```python
from build123d import *

# Parameters (mm, degrees)
EXTRUDE_THIN1_DEPTH = 76.2


with BuildPart() as part:
    # Sketch1 → Extrude-Thin1 (new body)
    with BuildSketch(Plane.XY):
        with BuildLine():
            Line((-171.530725158, -169.540176263), (-57.207776809, -14.493356815))
            ThreePointArc((-57.207776809, -14.493356815), (-48.029088686, -5.258412911), (-36.568222458, 0.920668726))
            Line((-36.568222458, 0.920668726), (143.952557391, 66.301099815))
            ThreePointArc((143.952557391, 66.301099815), (253.095507904, 33.210999285), (252.264699452, -80.834816757))
            Line((252.264699452, -80.834816757), (229.469051384, -110.874685447))
            Line((229.469051384, -110.874685447), (226.93983158, -108.955395947))
            Line((226.93983158, -108.955395947), (249.735479648, -78.915527258))
            ThreePointArc((249.735479648, -78.915527258), (250.538594484, 31.328761583), (145.033742323, 63.315858762))
            Line((145.033742323, 63.315858762), (-35.487037526, -2.064572327))
            ThreePointArc((-35.487037526, -2.064572327), (-46.129270453, -7.80229099), (-54.652337995, -16.377596044))
            Line((-54.652337995, -16.377596044), (-168.975286345, -171.424415492))
            Line((-168.975286345, -171.424415492), (-171.530725158, -169.540176263))
        make_face()
    extrude(amount=EXTRUDE_THIN1_DEPTH)


solid = part.part
```
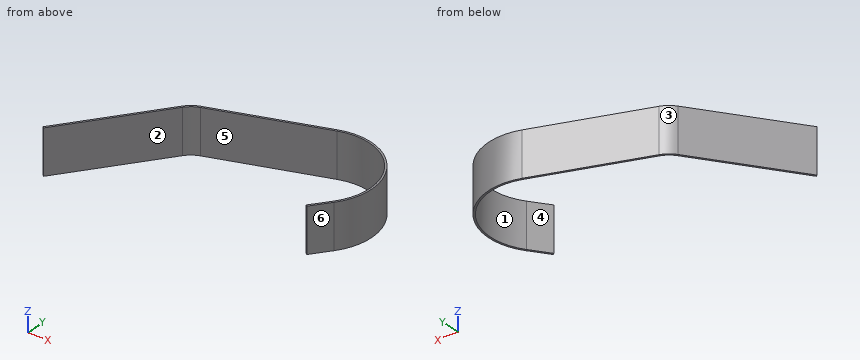
Design review of the part built by this model. Coordinates are the model's own, in mm. Face numbers are marked on the shaded views. A direction names the side the tool comes from. Round coordinates to 2 decimals unless told otherwise and drop trailing zeros. Order: outer loops, then holes, each group sorted by start corner. A loop starts at its lowest first (then second) coordinate and runs counter-clockwise, first axis right, second up. Notation, with made-up numbers: M -35.5,5 L -26.5,5 A17 cw -26.5,27 Z; hole C 20.5,63.25 d1. An arc over 180 degrees is marked long. Put each result on its own line as item: value.
Q1. To check wall thickness, follow line 1 (Y direction, x = 179, z = 57); line 2 (X direction, y = -25.5, z = 32.5); line 3 (X direction, y = -55.5, z = 34). State the ranges of each line that lie inside material, in increasing order.
Reported:
line 1: 68.78 to 71.96
line 2: -65.32 to -61.38, 268.44 to 271.61
line 3: -87.44 to -83.5, 262.63 to 266.01
Q2. Consider section D-D (y = -140). State the section outline as (x, z) points, and give its area (3 significant figures).
Reported:
outline: M -149.75,0 L -145.8,0 L -145.8,76.2 L -149.75,76.2 Z
area: 301 mm²
Q3. Draft analysis for pull direction Y (two halves, no side actions). For the marked faces 1, 2, 3 and 4, state which applies: released by +Y, released by -Y, zero draft, split by the parting line, or undercut.
Reported:
face 1: undercut
face 2: released by -Y
face 3: released by +Y
face 4: undercut
Q4. Consider section C-C (x = -48). State the section outline as (y, z) points.
Reported:
outline: M -9.29,0 L -5.24,0 L -5.24,76.2 L -9.29,76.2 Z
Q5. Insertion check: pin 1 Ø2 at (x, z) = (198, 55.5) entering from +Y; pin 2 Ø8 at (x, z) = (-93, 26.5) entering from -Y; pin 3 Ø3 at (x, z) = (208, 20) entering from +Y. Each pin has a flat end and moves straight along its axis. Give the tip position at first contact, or say it passes through.
Reported:
pin 1: y = 69.74
pin 2: y = -73.81
pin 3: y = 67.11
Q6. Machinability: for the marked faces 5 and 6, which of the approach directions +Z, -Z, +X, -X, +Y, -Y give a long, thin tool a straight path to every point of the face, cutting with its end or side? Answer none if there is none.
Reported:
face 5: +Z, -Z, -Y
face 6: +Z, -Z, +X, -Y
Q7. Consider section A-A (y = -59). State the section outline as (x, z) points, and give its area (3 significant figures).
Reported:
outline: M -90.02,0 L -86.08,0 L -86.08,76.2 L -90.02,76.2 Z; M 261.24,0 L 264.68,0 L 264.68,76.2 L 261.24,76.2 Z
area: 562 mm²
Q8. Consider section B-B (z = 41.5). State the section outline as (x, y) points (3 decimals).
Reported:
outline: M -171.531,-169.54 L -168.975,-171.424 L -54.652,-16.378 A41.275 cw -35.487,-2.065 L 145.034,63.316 A92.075 cw 249.735,-78.916 L 226.94,-108.955 L 229.469,-110.875 L 252.265,-80.835 A95.25 ccw 143.953,66.301 L -36.568,0.921 A44.45 ccw -57.208,-14.493 Z
